Could you check a few things on this model? Use its own coordinates, in mm. A direction names the side the tool comes from. Round coordinates to 2 decimals unless told otherwise and drop trailing zeros. Write each loop counter-clockwise with the first axis right and the second up, starting at its lowest first coordinate (ties: lowest second). Pieces come first, ordered by that corner, then holes. Notation, with made-up numbers: (-7, 68) -> (17, 68) arc R17 cw to (17, 82) -> close; hole circle Ø4 at (-0.5, 79). An arc over 180 degrees is marked (long way). Return JSON: item names as keys, results as strings.
Autodesk Inventor part; units mm, degrees
ref_plane "YZ Plane" through (0, 0, 0) normal (1, 0, 0) x (0, 1, 0)
ref_plane "XZ Plane" through (0, 0, 0) normal (0, 1, 0) x (-1, 0, 0)
ref_plane "XY Plane" through (0, 0, 0) normal (0, 0, 1) x (1, 0, 0)
sketch "스케치1" plane through (0, 0, 0) normal (0, 0, 1) x (1, 0, 0)
  line L0 (54.3328, -36.1894) -> (-54.3328, -36.1894)
  line L1 (-54.3328, -36.1894) -> (-54.3328, 36.1894)
  line L2 (-54.3328, 36.1894) -> (54.3328, 36.1894)
  line L3 (54.3328, 36.1894) -> (54.3328, -36.1894)
  line L4 (54.3328, -36.1894) -> (-54.3328, 36.1894) construction
  line L5 (-54.3328, -36.1894) -> (54.3328, 36.1894) construction
  point P0 (0, 0)
extrude "돌출1" add sketch "스케치1" along normal blind 70
sketch "스케치2" plane through (-54.3328, 36.1894, 0) normal (0, 1, 0) x (1, 0, 0)
  line L0 (0, -70) -> (108.6655, -70)
  line L1 (108.6655, 0) -> (0, 0)
  line L2 (29.224, -70) -> (66.7649, -70)
  line L3 (66.7649, -70) -> (66.7649, 0)
  line L4 (66.7649, 0) -> (29.224, 0)
  line L5 (29.224, 0) -> (29.224, -70)
  line L6 (66.7649, -52.0222) -> (98.3413, -52.0222)
  line L7 (98.3413, -52.0222) -> (98.3413, -16.2356)
  line L8 (98.3413, -16.2356) -> (66.7649, -16.2356)
  line L9 (66.7649, -16.2356) -> (66.7649, -52.0222)
  point P0 (54.3328, 0)
extrude "돌출2" cut sketch "스케치2" against normal blind 30 contours L5 L1 L3 L0
sketch "스케치3" plane through (54.3328, 36.1894, 70) normal (0, 1, 0) x (1, 0, 0)
  line L0 (-41.9007, 70) -> (-41.9007, 0)
  line L1 (0, 70) -> (0, 0)
  line L2 (-41.9007, 53.9806) -> (0, 53.9806)
  line L3 (0, 53.9806) -> (0, 17.7133)
  line L4 (0, 17.7133) -> (-41.9007, 17.7133)
  line L5 (-41.9007, 17.7133) -> (-41.9007, 53.9806)
  point P0 (-54.3328, 70)
extrude "돌출3" cut sketch "스케치3" against normal blind 30
sketch "스케치4" plane through (0, 0, 70) normal (0, 0, 1) x (1, 0, 0)
  point P0 (0, 0)
sketch "스케치5" plane through (12.4321, 36.1894, 0) normal (0, 1, 0) x (1, 0, 0)
  line L0 (41.9007, 0) -> (41.9007, -16.0194)
  line L1 (0, 0) -> (41.9007, 0)
  line L2 (41.9007, 0) -> (41.9007, -16.0194)
  line L3 (41.9007, -16.0194) -> (0, -16.0194)
  line L4 (0, -16.0194) -> (0, 0)
  line L5 (41.9007, -70) -> (0, -70)
  line L6 (0, -52.2867) -> (41.9007, -52.2867)
  line L7 (41.9007, -52.2867) -> (41.9007, -70)
  line L8 (41.9007, -70) -> (0, -70)
  line L9 (0, -70) -> (0, -52.2867)
  point P0 (-12.4321, 0)
extrude "돌출4" cut sketch "스케치5" against normal blind 20 contours L0 L3 L4 L1
extrude "돌출5" cut sketch "스케치5" against normal blind 20 contours L5 L9 L6 L7
properties part number "240503_3Dsketch06"
1) Thinking about a two-plate mould opening in Z: for faces 4 (the face through (54.333, -10, 35)), 5 (the face through (-1, -8, 0)), 6 (the face through (33, 11, 16.019)), which applies, pulls with the +Z half, pulls with the -Z half, needs draft (parallel to the pull), parting line crosses it, or undercut?
Return value:
{"face 4": "needs draft", "face 5": "pulls with the -Z half", "face 6": "undercut"}
2) I want a section at B-B, the plane z = 63. Please give me the cut outline in (x, y), and give its area (3 significant figures).
Return value:
{"outline": "(-54.33, -36.19) -> (54.33, -36.19) -> (54.33, 16.19) -> (12.43, 16.19) -> (12.43, 6.19) -> (-25.11, 6.19) -> (-25.11, 36.19) -> (-54.33, 36.19) -> close", "area": "5,900 mm²"}
3) I want a section at A-A, the plane y = 10. Please give me the cut outline in (x, z), and give its area (3 significant figures).
Return value:
{"outline": "(-54.33, 0) -> (-25.11, 0) -> (-25.11, 70) -> (-54.33, 70) -> close; (12.43, 0) -> (54.33, 0) -> (54.33, 16.02) -> (12.43, 16.02) -> close; (12.43, 52.29) -> (54.33, 52.29) -> (54.33, 70) -> (12.43, 70) -> close", "area": "3,460 mm²"}
4) If I drill on probe 1 along X at (y, z) = (9.5, 58.5); probe 2 along X at (y, z) = (17.5, 5.5); probe 3 along Y at (x, z) = (4, 51), over which ranges is the centre line in solid material (lowest first)? Write a range as [from, to].
Return value:
{"probe 1": "[-54.33, -25.11], [12.43, 54.33]", "probe 2": "[-54.33, -25.11]", "probe 3": "[-36.19, 6.19]"}
5) For faces 1 (the face through (34, 11, 52.287)), 2 (the face through (12.432, 11, 8)), 3 (the face through (33, 16.189, 61)), which set-ups out of +Z, -Z, +X, -X, +Y, -Y let a thin tool reach every point of the face, with its end or its side?
Return value:
{"face 1": "+X, +Y", "face 2": "+Z, -Z, +Y", "face 3": "+Z, -Z, +X, +Y"}
6) Will these pins go through, and if not, where does the flat tip stop? pin 1 Ø2 at (x, z) = (24.5, 55) entering from +Y; pin 2 Ø9 at (y, z) = (26, 46.5) entering from +X.
Return value:
{"pin 1": "y = 16.19", "pin 2": "x = -25.11"}
7) I want a section at D-D, the plane y = 18. Please give me the cut outline in (x, z).
Return value:
{"outline": "(-54.33, 0) -> (-25.11, 0) -> (-25.11, 70) -> (-54.33, 70) -> close"}
8) I want a section at C-C, the plane x = 19. Please give me the cut outline in (y, z).
Return value:
{"outline": "(-36.19, 0) -> (16.19, 0) -> (16.19, 16.02) -> (6.19, 16.02) -> (6.19, 52.29) -> (16.19, 52.29) -> (16.19, 70) -> (-36.19, 70) -> close"}
